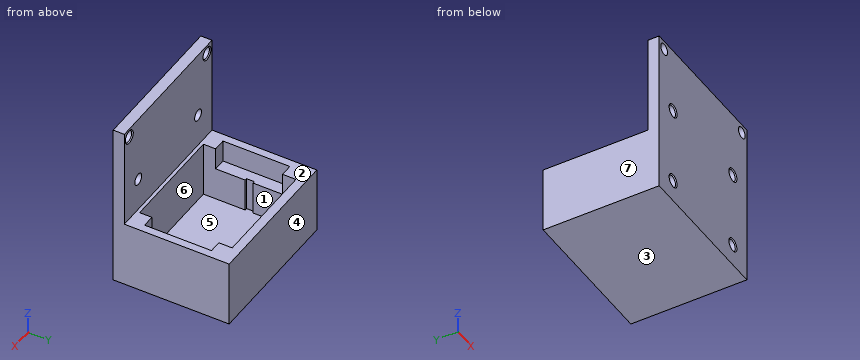
Autodesk Fusion 360 part; units mm, degrees
sketch "Sketch1" plane through (0, 0, 0) normal (0, 0, 1) x (1, 0, 0)
  line L0 (0, 0) -> (60, 0)
  line L1 (60, 0) -> (60, 50)
  line L2 (60, 50) -> (0, 50)
  line L3 (0, 50) -> (0, 0)
  dimension "d1" = 60
  dimension "d2" = 50
extrude "Extrude1" add sketch "Sketch1" along normal blind 30
sketch "Sketch2" plane through (0, 0, 30) normal (0, 0, 1) x (-1, 0, 0)
  line L0 (0, -50) -> (0, 0)
  line L1 (0, 0) -> (-60, 0)
  line L2 (-60, 0) -> (-60, -50)
  line L3 (-60, -50) -> (0, -50)
  line L4 (-54, -5) -> (-6, -5)
  line L5 (-6, -5) -> (-6, -45)
  line L6 (-6, -45) -> (-54, -45)
  line L7 (-54, -45) -> (-54, -5)
  line L8 (-54, -5) -> (-6, -45) construction
  line L9 (-6, -5) -> (-54, -45) construction
  point P0 (-30, -25)
  dimension "d5" = 48
  dimension "d6" = 40
extrude "Extrude2" cut sketch "Sketch2" against normal blind 25 contours L4 L5 L6 L7
sketch "Sketch3" plane through (0, 0, 30) normal (0, 0, 1) x (-1, 0, 0)
  line L0 (-6, -5) -> (-6, -45)
  line L1 (-6, -45) -> (-54, -45)
  line L2 (-54, -45) -> (-54, -5)
  line L3 (-54, -5) -> (-6, -5)
  line L4 (0, -50) -> (0, 0)
  line L5 (0, 0) -> (-60, 0)
  line L6 (-60, 0) -> (-60, -50)
  line L7 (-60, -50) -> (0, -50)
  line L8 (-54, -10) -> (-59.5, -10)
  line L9 (-59.5, -10) -> (-59.5, -40)
  line L10 (-59.5, -40) -> (-54, -40)
  line L11 (-54, -40) -> (-54, -10)
  line L12 (-6, -10) -> (-0.5, -10)
  line L13 (-0.5, -10) -> (-0.5, -40)
  line L14 (-0.5, -40) -> (-6, -40)
  line L15 (-6, -40) -> (-6, -10)
  dimension "d9" = 5.5
  dimension "d10" = 30
  dimension "d11" = 5.5
  dimension "d12" = 30
extrude "Extrude3" cut sketch "Sketch3" against normal blind 10 contours L0 L12 L13 L14 L15 | L2 L8 L9 L10 L11
move_face "OffsetFaces1" offset 3 1 faces at (0, 33.3333, 10)
move_face "OffsetFaces2" offset 3 1 faces at (60, 33.3333, 20)
move_face "OffsetFaces3" offset 2 1 faces at (19, 0, 20)
sketch "Sketch4" plane through (0, 0, 30) normal (0, 0, 1) x (-1, 0, 0)
  line L0 (-59.5, -10) -> (-54, -10)
  line L1 (-54, -10) -> (-54, -5)
  line L2 (-54, -5) -> (-6, -5)
  line L3 (-6, -5) -> (-6, -10)
  line L4 (-6, -10) -> (-0.5, -10)
  line L5 (-0.5, -10) -> (-0.5, -40)
  line L6 (-0.5, -40) -> (-6, -40)
  line L7 (-6, -40) -> (-6, -45)
  line L8 (-6, -45) -> (-54, -45)
  line L9 (-54, -45) -> (-54, -40)
  line L10 (-54, -40) -> (-59.5, -40)
  line L11 (-59.5, -40) -> (-59.5, -10)
  line L12 (3, -50) -> (3, 2)
  line L13 (3, 2) -> (-63, 2)
  line L14 (-63, 2) -> (-63, -50)
  line L15 (-63, -50) -> (3, -50)
  line L16 (3, 2) -> (-63, 2)
  line L17 (-63, 2) -> (-63, -3)
  line L18 (-63, -3) -> (3, -3)
  line L19 (3, -3) -> (3, 2)
  dimension "d18" = 66
  dimension "d19" = 5
extrude "Extrude4" add sketch "Sketch4" along normal blind 45 contours L12 L13 L14 L16 L17 L18 L19
sketch "Sketch7" plane through (0, 3, 0) normal (0, 1, 0) x (-1, 0, 0)
  line L0 (-63, 30) -> (3, 30)
  line L1 (3, 30) -> (3, 75)
  line L2 (3, 75) -> (-63, 75)
  line L3 (-63, 75) -> (-63, 30)
  point P0 (-59.25, 71)
  point P1 (-0.75, 71)
hole "Hole1" at (59.25, 3, 71) at (0.75, 3, 71) direction (0, -1, 0) diameter 5.1 depth 130 tip angle 118 countersink diameter 6 countersink angle 90
sketch "Sketch8" plane through (0, -2, 0) normal (0, -1, 0) x (1, 0, 0)
  circle A0 centre (59.25, 71) radius 2.55
  circle A1 centre (0.75, 71) radius 2.55
  line L0 (-3, 0) -> (63, 0)
  line L1 (63, 0) -> (63, 75)
  line L2 (63, 75) -> (-3, 75)
  line L3 (-3, 75) -> (-3, 0)
  point P0 (52.5, 45)
  point P1 (7.5, 45)
hole "Hole2" at (7.5, -2, 45) at (52.5, -2, 45) direction (0, 1, 0) diameter 5.1 depth 130 tip angle 118 countersink diameter 6 countersink angle 90
sketch "Sketch9" plane through (0, -2, 0) normal (0, -1, 0) x (1, 0, 0)
  circle A0 centre (7.5, 45) radius 3
  circle A1 centre (52.5, 45) radius 3
  circle A2 centre (59.25, 71) radius 2.55
  circle A3 centre (0.75, 71) radius 2.55
  line L0 (-3, 0) -> (63, 0)
  line L1 (63, 0) -> (63, 75)
  line L2 (63, 75) -> (-3, 75)
  line L3 (-3, 75) -> (-3, 0)
  point P0 (7.5, 10)
  point P1 (52.5, 10)
hole "Hole3" at (7.5, -2, 10) at (52.5, -2, 10) direction (0, 1, 0) diameter 5.1 depth 5.6 tip angle 180 countersink diameter 6 countersink angle 90
sketch "Sketch10" plane through (6, 0, 0) normal (1, 0, 0) x (0, 1, 0)
  line L0 (40, 30) -> (40, 20)
  line L1 (40, 20) -> (10, 20)
  line L2 (10, 20) -> (10, 30)
  line L3 (10, 30) -> (5, 30)
  line L4 (5, 30) -> (5, 5)
  line L5 (5, 5) -> (45, 5)
  line L6 (45, 5) -> (45, 30)
  line L7 (45, 30) -> (40, 30)
  line L8 (23.25, 30) -> (26.75, 30)
  line L9 (26.75, 30) -> (26.75, 0)
  line L10 (26.75, 0) -> (23.25, 0)
  line L11 (23.25, 0) -> (23.25, 30)
  point P0 (23.25, 30)
  dimension "d41" = 3.5
extrude "Extrude5" cut sketch "Sketch10" against normal blind 1 contours L1 L5 L9 L11
sketch "Sketch11" plane through (54, 0, 0) normal (-1, 0, 0) x (0, -1, 0)
  line L0 (-10, 30) -> (-10, 20)
  line L1 (-10, 20) -> (-40, 20)
  line L2 (-40, 20) -> (-40, 30)
  line L3 (-40, 30) -> (-45, 30)
  line L4 (-45, 30) -> (-45, 5)
  line L5 (-45, 5) -> (-5, 5)
  line L6 (-5, 5) -> (-5, 30)
  line L7 (-5, 30) -> (-10, 30)
  line L8 (-23.25, 30) -> (-26.75, 30)
  line L9 (-26.75, 30) -> (-26.75, 0)
  line L10 (-26.75, 0) -> (-23.25, 0)
  line L11 (-23.25, 0) -> (-23.25, 30)
  point P0 (-23.25, 30)
  dimension "d44" = 3.5
extrude "Extrude6" cut sketch "Sketch11" against normal blind 1 contours L1 L5 L9 L11
move_face "OffsetFaces4" offset -1 1 faces at (22, 45, 21.6667)
move_face "OffsetFaces5" offset -0.5 1 faces at (38, 5, 13.3333)
Geometry check sheet. Reference: the model listing, model coordinates, mm. Face numbers are marked on the shaded views. A direction names the side the tool comes from. Round coordinates to 2 decimals unless told otherwise and drop trailing zeros. Write each loop counter-clockwise with the first axis right and the second up, starting at its lowest first coordinate (ties: lowest second). Pieces come first, ordered by that corner, then holes. Notation, with made-up numbers: (34.5, 36) - (55.5, 36) arc R22 ccw to (55.5, 70) - close; hole circle Ø2 at (36, 39). An arc over 180 degrees is marked (long way). Write each question's results on one line, items separated by ' | '.
(1) Sectioned sample at C-C, the plane z = 28. Enter the section's corners in (x, y).
Computed:
outline: (-3, -2) - (63, -2) - (63, 50) - (-3, 50) - close; hole (0.5, 10) - (6, 10) - (6, 4.5) - (54, 4.5) - (54, 10) - (59.5, 10) - (59.5, 40) - (54, 40) - (54, 46) - (6, 46) - (6, 40) - (0.5, 40) - close
(2) Thickness scan on probe 1 along X at (y, z) = (0.35, 45); probe 2 along Z at (x, y) = (7.5, -0.45); probe 3 along X at (y, z) = (0.4, 71). Record the ranges inside material, lowest first. Write a range as from..to.
Computed:
probe 1: x = -3..4.95, 10.05..49.95, 55.05..63 | probe 2: z = 0..7.45, 12.55..42.45, 47.55..75 | probe 3: x = -3..-1.8, 3.3..56.7, 61.8..63
(3) Sectioned sample at D-D, the plane y = 5.5. Enter the section's corners in (x, z).
Computed:
outline: (-3, 0) - (63, 0) - (63, 30) - (54, 30) - (54, 5) - (6, 5) - (6, 30) - (-3, 30) - close
(4) Draft check along X on the marked faces 4, 5, 6 and 7. Enter one of: pulls with the +X half, pulls with the -X half, needs draft (parallel to the pull), parting line crosses it, or undercut.
Computed:
face 4: needs draft | face 5: undercut | face 6: undercut | face 7: pulls with the -X half
(5) Depth check by flat-ended pin: pin 1 Ø3 at (x, y) = (4.5, 27.5) entering from +Z; pin 2 Ø3 at (x, z) = (52.5, 10) entering from -Y; pin 3 Ø23.5 at (x, y) = (40.5, 16) entering from +Z. Enter the tip coordinate at first touch or a pass-through.
Computed:
pin 1: stops at z = 20 | pin 2: stops at y = 3.6 | pin 3: stops at z = 30
(6) Sectioned sample at B-B, the plane x = 52.5. Enter the section's corners in (y, z).
Computed:
outline: (-2, 0) - (50, 0) - (50, 30) - (46, 30) - (46, 5) - (4.5, 5) - (4.5, 30) - (3, 30) - (3, 42.45) - (-1.55, 42.45) - (-2, 42) - (-2, 13) - (-1.55, 12.55) - (3.6, 12.55) - (3.6, 7.45) - (-1.55, 7.45) - (-2, 7) - close; (-2, 48) - (-1.55, 47.55) - (3, 47.55) - (3, 75) - (-2, 75) - close
(7) Sectioned sample at A-A, the plane z = 71. Enter the section's corners in (x, y).
Computed:
outline: (-3, -2) - (-1.8, -2) - (-1.8, 2.55) - (-2.25, 3) - (-3, 3) - close; (3.3, -2) - (56.7, -2) - (56.7, 2.55) - (56.25, 3) - (3.75, 3) - (3.3, 2.55) - close; (61.8, -2) - (63, -2) - (63, 3) - (62.25, 3) - (61.8, 2.55) - close
(8) Set-up check for the marked faces 1, 2 and 3: record each of +Z, -Z, +X, -X, +Y, -Y from which the full face is reachable in a straight line by a thin tool's end or side.
Computed:
face 1: +Z | face 2: +Z, +X, -X, +Y | face 3: -Z, +X, -X, +Y, -Y
